Job drawing, mm, ordinate dimensions from the low corner. One solid piece. A direction names the side the tool comes from. Coordinates: 2 decimals unless noted, no trailing zeros. Order: outer loops, then holes, each group sorted by start corner. A loop starts at its lowest first (then second) coordinate and runs counter-clockwise, first axis right, second up. Notation, with made-up numbers: (23.5, 23) - (27.5, 23) arc R15 ccw to (27.5, 27) - close; hole circle Ø11 at (67.25, 66.25). An arc over 180 degrees is marked (long way). Use a Markdown table: item, result. Add a question column.
1) Saw through at A-A on z = 15. List the corners of the cut face in (x, y).
2) Saw through at B-B on x = 143.35. List the corners of the cut face in (y, z), then the cut area to 3 significant figures.
3) Tool access for the marked faces 1, 2 and 3: list every direction of +Z, -Z, +X, -X, +Y, -Y with a clear straight run to the whole face (end or side of a thin tool).
4) Saw through at D-D on z = 3.25. List the corners of the cut face in (x, y).
5) Drop flat-ended pins along their axis: P1, Ø12.5, axis at y = 16.5, z = 19.5, coming from the +X side; P2, Ø7.5, axis at x = 10.5, z = 15, coming from the +Y side; P3, Ø7.5, axis at y = 14, z = 10, coming from the -X side; P4, Ø5, axis at y = 4.5, z = 25.5, coming from the -X side. Give the stop position or say it passes through.
6) Wall check: L1, parallel to X at y = 1.55, z = 15; L2, parallel to X at y = 16, z = 24.25; L3, parallel to X at y = 3, z = 9.5. Give the ranges that are in metal, low to high. Write a range as [from, to].
7) Saw through at C-C on y = 23. List the corners of the cut face in (x, z).
8) Two-plate mould, pull along X, no slides. Class the marked faces 4, 5 and 6: +X half, -X half, draft (parallel to the pull), parting line (faces both ways), or undercut.
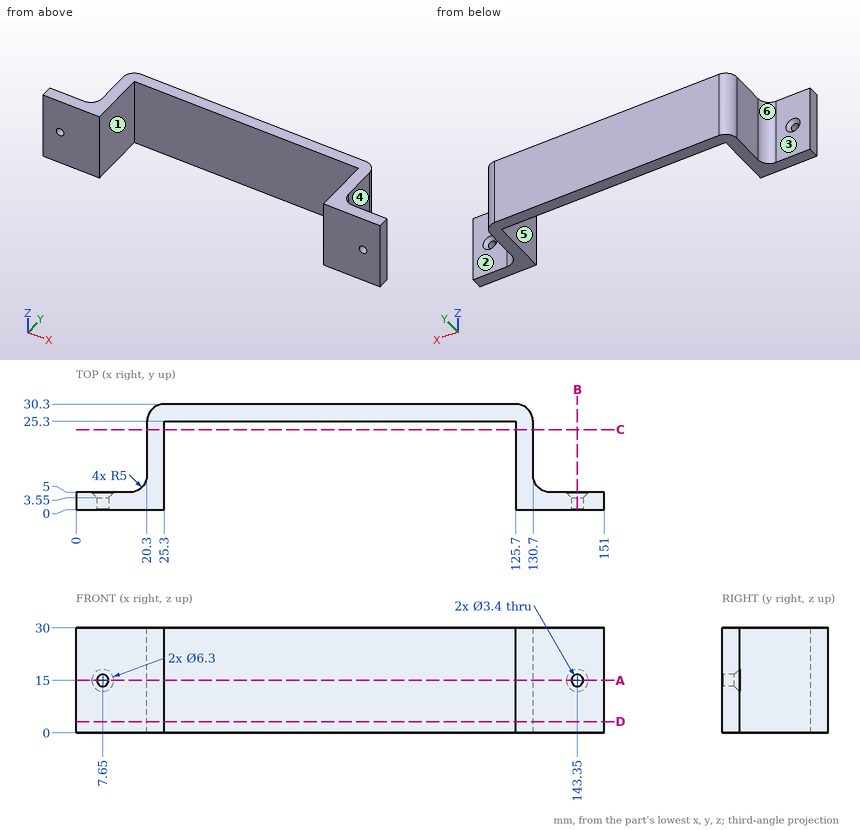
Results are:
| question | item | result |
|---|---|---|
| 1 | outline | (0, 0) - (5.95, 0) - (5.95, 3.55) - (4.5, 5) - (0, 5) - close; (9.35, 0) - (25.3, 0) - (25.3, 25.3) - (125.7, 25.3) - (125.7, 0) - (141.65, 0) - (141.65, 3.55) - (140.2, 5) - (135.7, 5) arc R5 cw to (130.7, 10) - (130.7, 25.3) arc R5 ccw to (125.7, 30.3) - (25.3, 30.3) arc R5 ccw to (20.3, 25.3) - (20.3, 10) arc R5 cw to (15.3, 5) - (10.8, 5) - (9.35, 3.55) - close; (145.05, 0) - (151, 0) - (151, 5) - (146.5, 5) - (145.05, 3.55) - close |
| 2 | outline | (0, 0) - (5, 0) - (5, 11.85) - (3.55, 13.3) - (0, 13.3) - close; (0, 16.7) - (3.55, 16.7) - (5, 18.15) - (5, 30) - (0, 30) - close |
| 2 | area | 131 mm2 |
| 3 | face 1 | +Z, -Z, -Y |
| 3 | face 2 | +Z, -Z, +X, +Y |
| 3 | face 3 | +Z, -Z, -X, +Y |
| 4 | outline | (0, 0) - (25.3, 0) - (25.3, 25.3) - (125.7, 25.3) - (125.7, 0) - (151, 0) - (151, 5) - (135.7, 5) arc R5 cw to (130.7, 10) - (130.7, 25.3) arc R5 ccw to (125.7, 30.3) - (25.3, 30.3) arc R5 ccw to (20.3, 25.3) - (20.3, 10) arc R5 cw to (15.3, 5) - (0, 5) - close |
| 5 | P1 | x = 130.7 |
| 5 | P2 | y = 5 |
| 5 | P3 | x = 20.3 |
| 5 | P4 | x = 0 |
| 6 | L1 | [0, 5.95], [9.35, 25.3], [125.7, 141.65], [145.05, 151] |
| 6 | L2 | [20.3, 25.3], [125.7, 130.7] |
| 6 | L3 | [0, 25.3], [125.7, 151] |
| 7 | outline | (20.3, 0) - (25.3, 0) - (25.3, 30) - (20.3, 30) - close; (125.7, 0) - (130.7, 0) - (130.7, 30) - (125.7, 30) - close |
| 8 | face 4 | +X half |
| 8 | face 5 | undercut |
| 8 | face 6 | -X half |
